from build123d import *

# Parameters (mm, degrees)
SKETCH_1_W          = 155
SKETCH_1_H          = 45
SKETCH_1_R          = 2.1
EXTRUDE_1_DEPTH     = 4
SKETCH_2_W          = 65
SKETCH_2_H          = 25
CUT_EXTRUDE_1_DEPTH = 10
SKETCH_3_R          = 2.1
EXTRUDE_2_DEPTH     = 4
FILLET_1_R          = 3


with BuildPart() as part:
    # 草图1 → 凸台-拉伸1 (new body)
    with BuildSketch(Plane.XY):
        Rectangle(SKETCH_1_W, SKETCH_1_H)
        with Locations((-67.5, 15)):
            Circle(SKETCH_1_R, mode=Mode.SUBTRACT)
        with Locations((-67.5, -15)):
            Circle(SKETCH_1_R, mode=Mode.SUBTRACT)
        with Locations(Location((67.5, 15, 0), (0, 0, 180))):
            Circle(SKETCH_1_R, mode=Mode.SUBTRACT)
        with Locations(Location((67.5, -15, 0), (0, 0, 180))):
            Circle(SKETCH_1_R, mode=Mode.SUBTRACT)
        with Locations((-47.5, 15)):
            Circle(SKETCH_1_R, mode=Mode.SUBTRACT)
        with Locations((47.5, 15)):
            Circle(SKETCH_1_R, mode=Mode.SUBTRACT)
        with Locations((-47.5, -10)):
            Circle(SKETCH_1_R, mode=Mode.SUBTRACT)
        with Locations((47.5, -10)):
            Circle(SKETCH_1_R, mode=Mode.SUBTRACT)
    extrude(amount=EXTRUDE_1_DEPTH)

    # 草图2 → 切除-拉伸1 (cut)
    with BuildSketch(Plane.XY.offset(4)):
        Rectangle(SKETCH_2_W, SKETCH_2_H)
    extrude(amount=-CUT_EXTRUDE_1_DEPTH, mode=Mode.SUBTRACT)

    # 草图3 → 凸台-拉伸2 (add)
    # profile 1 of 2: a face of its own
    with BuildSketch(Plane.XY.offset(4)):
        Polygon((-77.5, 22.5), (-95.5, 22.5), (-95.5, -2.5), (-77.5, -22.5), align=None)
        with Locations((-82.5, 12.5)):
            Circle(SKETCH_3_R, mode=Mode.SUBTRACT)
        with Locations((-82.5, 2.5)):
            Circle(SKETCH_3_R, mode=Mode.SUBTRACT)
    # profile 2 of 2: a face of its own
    with BuildSketch(Plane.XY.offset(4)):
        Polygon((77.5, 22.5), (95.5, 22.5), (95.5, -2.5), (77.5, -22.5), align=None)
        with Locations(Location((82.5, 12.5, 0), (0, 0, 180))):
            Circle(SKETCH_3_R, mode=Mode.SUBTRACT)
        with Locations(Location((82.5, 2.5, 0), (0, 0, 180))):
            Circle(SKETCH_3_R, mode=Mode.SUBTRACT)
    extrude(amount=-EXTRUDE_2_DEPTH)

    # 圆角1
    fillet_1_edges = [part.edges().sort_by_distance(p)[0] for p in [
        (32.5, 12.5, 2),
        (32.5, -12.5, 2),
        (-32.5, -12.5, 2),
        (-32.5, 12.5, 2),
        (-95.5, -2.5, 2),
        (-95.5, 22.5, 2),
        (77.5, -22.5, 2),
        (-77.5, -22.5, 2),
        (95.5, 22.5, 2),
        (95.5, -2.5, 2),
    ]]
    fillet(fillet_1_edges, radius=FILLET_1_R)


solid = part.part
Geometry: final body of the model. Coordinates: model frame, mm. A direction names the side the tool comes from. Round coordinates to 2 decimals unless told otherwise and drop trailing zeros. Loops run counter-clockwise (first coordinate to the right, second up) from the corner with the lowest first, then second, coordinate; pieces in that order, holes last. Notation, with made-up numbers: (-21.75, -8.75) - (-11.75, -8.75) arc R37 ccw to (-11.75, 27.25) - close; hole circle Ø4 at (-4.5, 83). An arc over 180 degrees is marked (long way). Write each question's results on one line, items separated by ' | '. Start each with the question number.
1) Cut plane D-D on x = -47.5. Return loops of the section in (y, z).
2) Access query for faces 4 (the face through (0, 12.5, 2)), 5 (the face through (-1, 15, 0)). Directions: +Z, -Z, +X, -X, +Y, -Y. A direction counts if a zero-diameter tool reaches every point of the face in a straight line with its end or side. Return the directions, or none.
3) Cut plane A-A on x = -23.5. Return loops of the section in (y, z).
4) Line query: probe 1 along Y at (x, z) = (-47.5, 3); probe 2 along Y at (x, z) = (67.5, 1.75); probe 3 along X at (y, z) = (11.5, 0.55). Output: solid intervals per line, ascending. Write a range as [from, to].
5) Cut plane B-B on y = 2.5. Return loops of the section in (x, z).
6) Cut plane C-C on z = 1.85. Count the separate pieces of the cut face and the enclosed holes in it, then the cut area to 3 significant figures.
7) Mould query, pull axis X, two halves, no side actions, for faces 1 (the face through (95.5, 9, 2)), 2 (the face through (-95.5, 9, 2)), 3 (the face through (84.6, 2.41, 2.03)). Classes: released by +X, released by -X, zero draft, split by the parting line, or undercut.
Verdict:
1) outline: (-22.5, 0) - (-12.1, 0) - (-12.1, 4) - (-22.5, 4) - close; (-7.9, 0) - (12.9, 0) - (12.9, 4) - (-7.9, 4) - close; (17.1, 0) - (22.5, 0) - (22.5, 4) - (17.1, 4) - close
2) face 4: +Z, -Z | face 5: -Z, +X, -X, +Y, -Y
3) outline: (-22.5, 0) - (-12.5, 0) - (-12.5, 4) - (-22.5, 4) - close; (12.5, 0) - (22.5, 0) - (22.5, 4) - (12.5, 4) - close
4) probe 1: y = [-22.5, -12.1], [-7.9, 12.9], [17.1, 22.5] | probe 2: y = [-22.5, -17.1], [-12.9, 12.9], [17.1, 22.5] | probe 3: x = [-95.5, -84.35], [-80.65, -31.74], [31.74, 80.65], [84.35, 95.5]
5) outline: (-95.5, 0) - (-84.6, 0) - (-84.6, 4) - (-95.5, 4) - close; (-80.4, 0) - (-32.5, 0) - (-32.5, 4) - (-80.4, 4) - close; (32.5, 0) - (80.4, 0) - (80.4, 4) - (32.5, 4) - close; (84.6, 0) - (95.5, 0) - (95.5, 4) - (84.6, 4) - close
6) separate pieces: 1 | enclosed holes: 13 | area: 6,450 mm2
7) face 1: released by +X | face 2: released by -X | face 3: undercut
